```python
from build123d import *

# Parameters (mm, degrees)
F0_W     = 34.5
F0_H     = 41
F1_DEPTH = 28.1
F2_R     = 0.5
F3_DEPTH = 5
F4_W     = 34.5
F4_H     = 41
F4_W_2   = 24.5
F4_H_2   = 31
F5_DEPTH = 5
F6_R     = 1


with BuildPart() as f1:
    # F0 (on Top) → F1 (new body)
    with BuildSketch(Plane.XY):
        Rectangle(F0_W, F0_H)
    extrude(amount=F1_DEPTH)

    # F2 (on face) → F3 (join)
    with BuildSketch(Plane(origin=(0, 0, 0), x_dir=(1, 0, 0), z_dir=(0, 0, -1))):
        with Locations((-12.5, 10)):
            Circle(F2_R)
        with Locations((-12.5, -10)):
            Circle(F2_R)
        with Locations((12.5, 10)):
            Circle(F2_R)
        with Locations((12.5, -10)):
            Circle(F2_R)
        with Locations((12.5, -5)):
            Circle(F2_R)
        with Locations((12.5, 5)):
            Circle(F2_R)
    extrude(amount=F3_DEPTH)

    # F4 (on face) → F5 (cut)
    with BuildSketch(Plane.XY.offset(28.1)):
        Rectangle(F4_W, F4_H)
        Rectangle(F4_W_2, F4_H_2, mode=Mode.SUBTRACT)
    extrude(amount=-F5_DEPTH, mode=Mode.SUBTRACT)

    # F6
    f6_edges = [f1.edges().sort_by_distance(p)[0] for p in [
        (-12.25, 0, 28.1),
        (0, -15.5, 28.1),
        (12.25, 0, 28.1),
        (0, 15.5, 28.1),
        (17.25, -20.5, 11.55),
        (17.25, 20.5, 11.55),
        (-17.25, -20.5, 11.55),
        (0, -20.5, 23.1),
        (17.25, 0, 23.1),
        (0, 20.5, 23.1),
        (-17.25, 0, 23.1),
        (-17.25, 20.5, 11.55),
    ]]
    fillet(f6_edges, radius=F6_R)


solid = f1.part
```
Work out the finished part from the listing and answer in its coordinate system (mm). A direction names the side the tool comes from. Coordinates: 2 decimals unless noted, no trailing zeros. Write each loop counter-clockwise with the first axis right and the second up, starting at its lowest first coordinate (ties: lowest second). Pieces come first, ordered by that corner, then holes.
Q1. Find the intervals of material crossed by line 1 (Z direction, x = -13, y = 9); line 2 (Z direction, x = 0.5, y = 3); line 3 (X direction, y = -13, z = 24.5), in increasing order.
Q2. A cutting plane is placed at A-A, the plane z = -2. Give the vertices of the cut face in (x, y), then the cut area to 3 significant figures.
Q3. A cutting plane is placed at B-B, the plane y = -3. Give the vertices of the cut face in (x, z).
Q4. A cutting plane is placed at C-C, the plane x = 9. Give the vertices of the cut face in (y, z), then the cut area to 3 significant figures.
Q5. Which of the six approach directions +Z, -Z, +X, -X, +Y, -Y give full straight-line access (tool end or side, diameter ignored) to faces 1 (the face through (12.25, 0, 25)), 2 (the face through (0, -15.5, 25)), 3 (the face through (13, -10, -2))?
Q6. Each of these flat-tipped pins is pushed along its axis until it touches: pin 1 Ø4.5 at (y, z) = (3.5, 24.5) entering from +X; pin 2 Ø2 at (y, z) = (-4, 25) entering from -X; pin 3 Ø17 at (x, y) = (-1, -7) entering from -Z. Where does it stop, or does it pass through?
Q7. A cutting plane is placed at D-D, the plane z = 25. Give the vertices of the cut face in (x, y), then the cut area to 4 significant figures.
Findings below:
1. line 1: z = 0 to 23.1
1. line 2: z = 0 to 28.1
1. line 3: x = -12.25 to 12.25
2. outline: circle Ø1 at (-12.5, -10); circle Ø1 at (-12.5, 10); circle Ø1 at (12.5, -10); circle Ø1 at (12.5, -5); circle Ø1 at (12.5, 5); circle Ø1 at (12.5, 10)
2. area: 4.71 mm2
3. outline: (-17.25, 0) - (17.25, 0) - (17.25, 22.1) arc R1 ccw to (16.25, 23.1) - (12.25, 23.1) - (12.25, 27.1) arc R1 ccw to (11.25, 28.1) - (-11.25, 28.1) arc R1 ccw to (-12.25, 27.1) - (-12.25, 23.1) - (-16.25, 23.1) arc R1 ccw to (-17.25, 22.1) - close
4. outline: (-20.5, 0) - (20.5, 0) - (20.5, 22.1) arc R1 ccw to (19.5, 23.1) - (15.5, 23.1) - (15.5, 27.1) arc R1 ccw to (14.5, 28.1) - (-14.5, 28.1) arc R1 ccw to (-15.5, 27.1) - (-15.5, 23.1) - (-19.5, 23.1) arc R1 ccw to (-20.5, 22.1) - close
4. area: 1,100 mm2
5. face 1: +Z, +X, +Y, -Y
5. face 2: +Z, +X, -X, -Y
5. face 3: -Z
6. pin 1: stops at x = 17.24
6. pin 2: stops at x = -12.25
6. pin 3: stops at z = 0
7. outline: (-12.25, -15.5) - (12.25, -15.5) - (12.25, 15.5) - (-12.25, 15.5) - close
7. area: 759.5 mm2
